The model under review builds one solid part; all positions refer to its coordinate system, in mm. Face numbers are marked on the shaded views. Give positions to 0.01 mm unless a question says otherwise; leave off trailing zeros. Loops run counter-clockwise (first coordinate to the right, second up) from the corner with the lowest first, then second, coordinate; pieces in that order, holes last. Notation, with made-up numbers: (82, 62.5) - (140, 62.5) arc R21 ccw to (140, 93.5) - close; hole circle Ø1 at (27, 78.5). An arc over 180 degrees is marked (long way). Return JSON: item names as keys, results as strings. Group by question number.
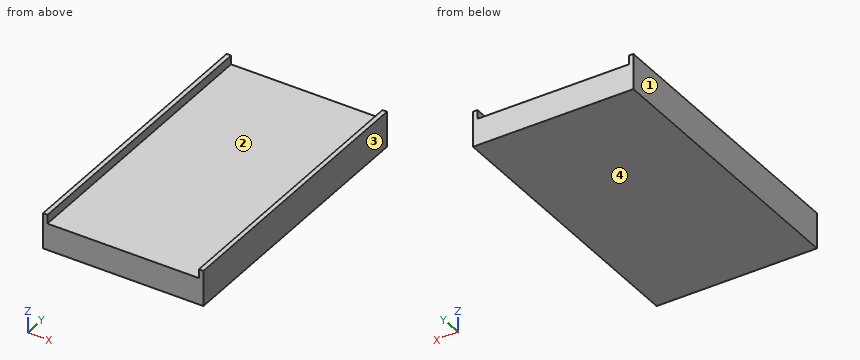
from build123d import *

# Parameters (mm, degrees)
SKETCH1_W           = 4.25
SKETCH1_H           = 8
BOSS_EXTRUDE1_DEPTH = 0.75
SKETCH1_3_W         = 0.125
SKETCH1_3_H         = 8
BOSS_EXTRUDE2_DEPTH = 1


with BuildPart() as part:
    # Sketch1 → Boss-Extrude1 (new body)
    with BuildSketch(Plane.XY):
        Rectangle(SKETCH1_W, SKETCH1_H)
    extrude(amount=BOSS_EXTRUDE1_DEPTH)

    # Sketch1<3> → Boss-Extrude2 (add)
    with BuildSketch(Plane.XY):
        with Locations((2.1875, 0)):
            Rectangle(SKETCH1_3_W, SKETCH1_3_H)
        with Locations((-2.1875, 0)):
            Rectangle(SKETCH1_3_W, SKETCH1_3_H)
    extrude(amount=BOSS_EXTRUDE2_DEPTH)


solid = part.part
Item 1: Take a section at C-C (x = 1.7). State the section outline as (y, z) points.
Item 2: Mouldability with a two-part tool opening along X and no side actions: class the marked faces 1, 2, 3 and 4 as +X half, -X half, draft (parallel to the pull), parting line (faces both ways), or undercut.
Item 3: Take a section at A-A (z = 0.9). State the section outline as (x, y) points (3 decimals).
Item 4: Take a section at B-B (y = -1.5). State the section outline as (x, z) points (3 decimals).
Item 5: For L1, parallel to Z at x = -1.4, y = 2.75, list the stretches that pass through material, from the lowest coordinate up. Write a range as from..to.
Check sheet entries:
{
 "1": {"outline": "(-4, 0) - (4, 0) - (4, 0.75) - (-4, 0.75) - close"},
 "2": {"face 1": "-X half", "face 2": "undercut", "face 3": "+X half", "face 4": "draft"},
 "3": {"outline": "(-2.25, -4) - (-2.125, -4) - (-2.125, 4) - (-2.25, 4) - close; (2.125, -4) - (2.25, -4) - (2.25, 4) - (2.125, 4) - close"},
 "4": {"outline": "(-2.25, 0) - (2.25, 0) - (2.25, 1) - (2.125, 1) - (2.125, 0.75) - (-2.125, 0.75) - (-2.125, 1) - (-2.25, 1) - close"},
 "5": {"L1": "z = 0..0.75"}
}
